Geometry check sheet. Reference: the model listing, model coordinates, mm. A direction names the side the tool comes from. Coordinates: 2 decimals unless noted, no trailing zeros. Write each loop counter-clockwise with the first axis right and the second up, starting at its lowest first coordinate (ties: lowest second). Pieces come first, ordered by that corner, then holes. Notation, with made-up numbers: (73.25, -3.75) -> (100.25, -3.75) arc R9 ccw to (100.25, 5.25) -> close; hole circle Ø6 at (58.5, 43.5). An arc over 180 degrees is marked (long way). Use a Markdown table: item, result.
```python
from build123d import *

# Parameters (mm, degrees)
RESSALTO_EXTRUS_O1_DEPTH = 5
ESBO_O2_W                = 71.017341725
ESBO_O2_H                = 15.188699459
CORTE_EXTRUS_O1_DEPTH    = 3
MOVER_FACE1_BY           = 10.718934909
ESBO_O3_W                = 68.089828176
ESBO_O3_H                = 2.204794608
CORTE_EXTRUS_O2_DEPTH    = 10
ESBO_O4_W                = 20.131000956
ESBO_O4_H                = 20.074327354
ESBO_O4_W_2              = 27.282150264
ESBO_O4_H_2              = 55.406342203
CORTE_EXTRUS_O4_DEPTH    = 1
ESBO_O5_R                = 1.188185025
ESBO_O5_R_2              = 1.258078261
ESBO_O5_R_3              = 1.220632904
CORTE_EXTRUS_O5_DEPTH    = 10
ESBO_O6_W                = 25.148684125
ESBO_O6_H                = 11.582759477
ESBO_O6_W_2              = 25.779007711
RESSALTO_EXTRUS_O2_DEPTH = 10
ESBO_O7_W                = 10
ESBO_O7_H                = 9.769511044
CORTE_EXTRUS_O7_DEPTH    = 99


with BuildPart() as part:
    # Esboço1 → Ressalto-extrusão1 (new body)
    with BuildSketch(Plane.XY):
        Polygon((-44.67348187, 40.715072084), (-44.67348187, 19.603553226), (-9.047793796, 19.603553226), (-9.047793796, 9.424785205), (-44.67348187, 9.424785205), (-44.67348187, -71.439871851), (45.61596039, -71.439871851), (45.61596039, 9.424785205), (10.178768021, 9.424785205), (10.178768021, 19.603553226), (45.61596039, 19.603553226), (45.61596039, 40.715072084), align=None)
    extrude(amount=RESSALTO_EXTRUS_O1_DEPTH)

    # Esboço2 → Corte-extrusão1 (cut)
    with BuildSketch(Plane.XY.offset(5)):
        with Locations((0.47123926, 33.120722355)):
            Rectangle(ESBO_O2_W, ESBO_O2_H)
    extrude(amount=-CORTE_EXTRUS_O1_DEPTH, mode=Mode.SUBTRACT)

    # Mover face1: a face moved outward by 10.718935
    extrude(part.faces().sort_by_distance((0.47123926, -71.439871851, 2.5))[0], amount=MOVER_FACE1_BY, dir=(0, -1, 0))

    # Esboço3 → Corte-extrusão2 (cut)
    with BuildSketch(Plane.XY.offset(2)):
        with Locations((0.67810757, 38.709026673)):
            Rectangle(ESBO_O3_W, ESBO_O3_H)
    extrude(amount=-CORTE_EXTRUS_O2_DEPTH, mode=Mode.SUBTRACT)

    # Esboço4 → Corte-extrusão4 (cut)
    with BuildSketch(Plane.XY.offset(5)):
        with Locations((0.001720335, -69.421605448)):
            Rectangle(ESBO_O4_W, ESBO_O4_H)
        with Locations((0.003895482, -25.35309655)):
            Rectangle(ESBO_O4_W_2, ESBO_O4_H_2)
    extrude(amount=-CORTE_EXTRUS_O4_DEPTH, mode=Mode.SUBTRACT)

    # Esboço5 → Corte-extrusão5 (cut)
    with BuildSketch(Plane(origin=(0, 0, 0), x_dir=(-1, 0, 0), z_dir=(0, 0, -1))):
        with Locations((-8.517583176, -50.2919249)):
            Circle(ESBO_O5_R)
        with Locations((-8.517583176, -64.550145197)):
            Circle(ESBO_O5_R_2)
        with Locations((8.885832774, -64.550145197)):
            Circle(ESBO_O5_R_3)
        with Locations((8.885832774, -50.2919249)):
            Circle(ESBO_O5_R)
    extrude(amount=-CORTE_EXTRUS_O5_DEPTH, mode=Mode.SUBTRACT)

    # Esboço6 → Ressalto-extrusão2 (add)
    with BuildSketch(Plane.XY.offset(5)):
        with Locations((33.041618328, -39.175755318)):
            Rectangle(ESBO_O6_W, ESBO_O6_H)
        with Locations((-31.783978015, -39.175755318)):
            Rectangle(ESBO_O6_W_2, ESBO_O6_H)
    extrude(amount=RESSALTO_EXTRUS_O2_DEPTH)

    # Esboço7 → Corte-extrusão7 (cut)
    with BuildSketch(Plane(origin=(45.61596039, 0, 0), x_dir=(0, 0, -1), z_dir=(1, 0, 0))):
        with Locations((-10, -39.181904772)):
            Rectangle(ESBO_O7_W, ESBO_O7_H)
    extrude(amount=-CORTE_EXTRUS_O7_DEPTH, mode=Mode.SUBTRACT)


solid = part.part
```
Item 1: Section check A-A on x = 16.5. Record the boundary of the cut face in (y, z).
Answer block:
| item | result |
|---|---|
| outline | (-82.16, 0) -> (9.42, 0) -> (9.42, 5) -> (-82.16, 5) -> close; (19.6, 0) -> (37.61, 0) -> (37.61, 2) -> (25.53, 2) -> (25.53, 5) -> (19.6, 5) -> close; (39.81, 0) -> (40.72, 0) -> (40.72, 2) -> (39.81, 2) -> close |
Item 2: Thickness scan on L1, parallel to Y at x = 21, z = 10.5; L2, parallel to X at y = -65, z = 1.75; L3, parallel to X at y = 30, z = 2.75. Record the ranges inside material, lowest first. Write a range as [from, to].
Answer block:
| item | result |
|---|---|
| L1 | y = [-44.97, -44.07], [-34.3, -33.38] |
| L2 | x = [-44.67, -10.02], [-7.75, 7.34], [9.69, 45.62] |
| L3 | x = [-44.67, -35.04], [35.98, 45.62] |
Item 3: Section check C-C on x = 5. Record the boundary of the cut face in (y, z), then the cut area to 3 significant figures.
Answer block:
| item | result |
|---|---|
| outline | (-82.16, 0) -> (37.61, 0) -> (37.61, 2) -> (25.53, 2) -> (25.53, 5) -> (2.35, 5) -> (2.35, 4) -> (-53.06, 4) -> (-53.06, 5) -> (-59.38, 5) -> (-59.38, 4) -> (-79.46, 4) -> (-79.46, 5) -> (-82.16, 5) -> close; (39.81, 0) -> (40.72, 0) -> (40.72, 2) -> (39.81, 2) -> close |
| area | 489 mm^2 |
Item 4: Mould release check, pull along Y, two halves, no side actions. Record for faces 4 (the flat face through (-9.048, 15, 2)), 5 (the flat face through (-27, 9.425, 2)), 6 (the flat face through (45.616, 30, 2)), 7 (the flat face through (33, -44.967, 10)): +Y half, -Y half, draft (parallel to the pull), parting line (faces both ways), or undercut.
Answer block:
| item | result |
|---|---|
| face 4 | undercut |
| face 5 | undercut |
| face 6 | draft |
| face 7 | -Y half |
Item 5: Depth check by flat-ended pin: P1, Ø3, axis at x = -8.89, y = -64.55, coming from the -Z side; P2, Ø2.5, axis at y = 15.5, z = 2.5, coming from the +X side; P3, Ø22, axis at x = 3.5, y = -74, coming from the +Z side; P4, Ø5, axis at x = -25.5, z = 10.5, coming from the +Y side. Enter the tip coordinate at first touch or a pass-through.
Answer block:
| item | result |
|---|---|
| P1 | stops at z = 0 |
| P2 | stops at x = 10.18 |
| P3 | stops at z = 5 |
| P4 | stops at y = -33.38 |
Item 6: Tool access check on faces 1 (the flat face through (33, -44.067, 10)), 2 (the flat face through (-32, -33.384, 10)), 3 (the flat face through (35.98, 33, 4)). Record the directions out of +Z, -Z, +X, -X, +Y, -Y that give a thin tool (end or side, any length) a straight path to the whole face; none if there is none.
Answer block:
| item | result |
|---|---|
| face 1 | +Z, +X, -X |
| face 2 | +Z, +X, -X, +Y |
| face 3 | +Z, +Y |
Item 7: Section check B-B on z = 10.5. Record the boundary of the cut face in (x, y), then the cut area to 3 significant figures.
Answer block:
| item | result |
|---|---|
| outline | (-44.67, -44.97) -> (-18.89, -44.97) -> (-18.89, -44.07) -> (-44.67, -44.07) -> close; (-44.67, -34.3) -> (-18.89, -34.3) -> (-18.89, -33.38) -> (-44.67, -33.38) -> close; (20.47, -44.97) -> (45.62, -44.97) -> (45.62, -44.07) -> (20.47, -44.07) -> close; (20.47, -34.3) -> (45.62, -34.3) -> (45.62, -33.38) -> (20.47, -33.38) -> close |
| area | 92.3 mm^2 |
Item 8: Section check D-D on y = -24. Record the boundary of the cut face in (x, z), then the cut area to 3 significant figures.
Answer block:
| item | result |
|---|---|
| outline | (-44.67, 0) -> (45.62, 0) -> (45.62, 5) -> (13.64, 5) -> (13.64, 4) -> (-13.64, 4) -> (-13.64, 5) -> (-44.67, 5) -> close |
| area | 424 mm^2 |
